from build123d import *

# Parameters (mm, degrees)
HUB_SKETCH_R              = 2.5
HUB_DEPTH                 = 3
POINTER_DEPTH             = 0.8
TAIL_SKETCH_W             = 7.1
TAIL_SKETCH_H             = 3
TAIL_DEPTH                = 3
TAIL_END_SKETCH_R         = 1.5
TAIL_END_DEPTH            = 3
SHAFT_BORE_DEPTH          = 23.343902972
SHAFT_BORE_DEPTH_BACK     = 23.343902972
BORE_SKETCH_R             = 1
SET_SCREW_HOLE_DEPTH      = 23.343902972
SET_SCREW_HOLE_DEPTH_BACK = 23.343902972
SETSCREW_SKETCH_R         = 0.6


with BuildPart() as part:
    # HUB_SKETCH → HUB (new body)
    with BuildSketch(Plane(origin=(0, 0, 0), x_dir=(1, 0, 0), z_dir=(0, 1, 0))):
        with Locations(Location((0, 0, 0), (0, 0, 270))):
            Circle(HUB_SKETCH_R)
    extrude(amount=HUB_DEPTH)

    # POINTER_SKETCH → POINTER (add)
    with BuildSketch(Plane(origin=(0, 0, 0), x_dir=(1, 0, 0), z_dir=(0, 1, 0))):
        Polygon((2, 1.5), (22, 0.3), (22, -0.3), (2, -1.5), align=None)
    extrude(amount=POINTER_DEPTH)

    # TAIL_SKETCH → TAIL (add)
    with BuildSketch(Plane(origin=(0, 0, 0), x_dir=(1, 0, 0), z_dir=(0, 1, 0))):
        with Locations((-3.55, 0)):
            Rectangle(TAIL_SKETCH_W, TAIL_SKETCH_H)
    extrude(amount=TAIL_DEPTH)

    # TAIL_END_SKETCH → TAIL_END (add)
    with BuildSketch(Plane(origin=(0, 0, 0), x_dir=(1, 0, 0), z_dir=(0, 1, 0))):
        with Locations((-7.1, 0)):
            Circle(TAIL_END_SKETCH_R)
    extrude(amount=TAIL_END_DEPTH)

    # BORE_SKETCH → SHAFT_BORE (cut, two sides: drawn at the far end of the back side and taken through both)
    with BuildSketch(Plane(origin=(0, 0, 0), x_dir=(1, 0, 0), z_dir=(0, 1, 0)).offset(-SHAFT_BORE_DEPTH_BACK)):
        with Locations(Location((0, 0, 0), (0, 0, 270))):
            Circle(BORE_SKETCH_R)
    extrude(amount=SHAFT_BORE_DEPTH + SHAFT_BORE_DEPTH_BACK, mode=Mode.SUBTRACT)

    # SETSCREW_SKETCH → SET_SCREW_HOLE (cut, two sides: drawn at the far end of the back side and taken through both)
    with BuildSketch(Plane.XY.offset(-SET_SCREW_HOLE_DEPTH_BACK)):
        with Locations((0, 1.46538664)):
            Circle(SETSCREW_SKETCH_R)
    extrude(amount=SET_SCREW_HOLE_DEPTH + SET_SCREW_HOLE_DEPTH_BACK, mode=Mode.SUBTRACT)


solid = part.part
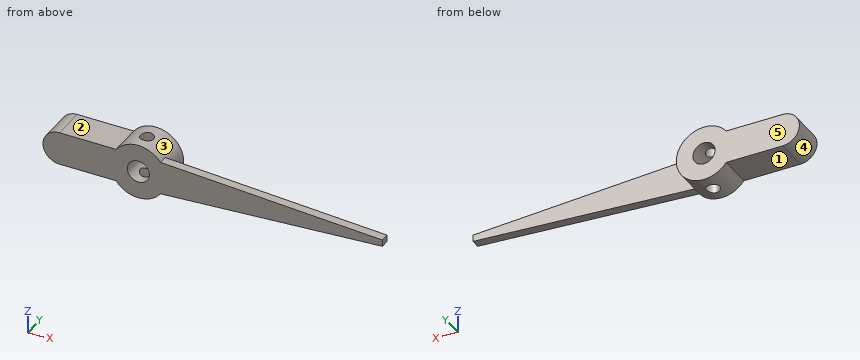
The model under review builds one solid part; all positions refer to its coordinate system, in mm. Face numbers are marked on the shaded views. A direction names the side the tool comes from. Round coordinates to 2 decimals unless told otherwise and drop trailing zeros. Order: outer loops, then holes, each group sorted by start corner. A loop starts at its lowest first (then second) coordinate and runs counter-clockwise, first axis right, second up. Notation, with made-up numbers: (85, 60) - (139, 60) arc R24 cw to (139, 84) - close; hole circle Ø5 at (62, -36.75). An arc over 180 degrees is marked (long way). Use one line per item in the form item = value.
Q1. Add section B-B on z = 0. Give the boundary of the cut face in (x, y), then the cut area to 3 significant figures.
Response values:
outline = (-8.6, 0) - (-1, 0) - (-1, 3) - (-8.6, 3) - close; (1, 0) - (22, 0) - (22, 0.8) - (2.5, 0.8) - (2.5, 3) - (1, 3) - close
area = 42.9 mm^2
Q2. Tool access review of the marked faces 1, 2, 3, 4 and 5: name each direction out of +Z, -Z, +X, -X, +Y, -Y from which nothing blocks a thin tool from reaching the whole face with its end or side.
Response values:
face_1 = -Z, -X, +Y, -Y
face_2 = +Z, -X, +Y, -Y
face_3 = +Y
face_4 = -X, +Y, -Y
face_5 = +Z, -Z, +X, -X, +Y
Q3. To check wall thickness, follow line 1 (Y direction, x = 0, z = -1.4); line 2 (X direction, y = 1.05, z = 0); line 3 (X direction, y = 0.4, z = -0.05). State the ranges of each line that lie inside material, in increasing order.
Response values:
line_1 = 0 to 0.87, 2.07 to 3
line_2 = -8.6 to -1, 1 to 2.5
line_3 = -8.6 to -1, 1 to 22
Q4. Clearance check with flat-ended pins moving along their axes: P1, Ø1.5, axis at y = 2.5, z = -1, coming from the +X side; P2, Ø1.1, axis at x = 0, y = 1.47, coming from the +Z side; P3, Ø1.5, axis at x = 13, z = 0, coming from the +Y side. State where each tip first meets the part, or that it passes through.
Response values:
P1 = 2.49
P2 = through
P3 = 0.8
Q5. Add section D-D on z = 1.85. Give the boundary of the cut face in (x, y), then the cut area to 3 significant figures.
Response values:
outline = (-1.68, 0) - (1.68, 0) - (1.68, 3) - (-1.68, 3) - close; hole circle Ø1.2 at (0, 1.47)
area = 8.96 mm^2
Q6. Add section A-A on x = 0. Give the boundary of the cut face in (y, z), then the cut area to 3 significant figures.
Response values:
outline = (0, -2.5) - (0.87, -2.5) - (0.87, -1) - (0, -1) - close; (0, 1) - (0.87, 1) - (0.87, 2.5) - (0, 2.5) - close; (2.07, -2.5) - (3, -2.5) - (3, -1) - (2.07, -1) - close; (2.07, 1) - (3, 1) - (3, 2.5) - (2.07, 2.5) - close
area = 5.40 mm^2
Q7. Add section C-C on y = 0.5. Give the boundary of the cut face in (x, z), then the cut area to 3 significant figures.
Response values:
outline = (-7.1, -1.5) - (-2, -1.5) arc R2.5 ccw to (2, -1.5) - (22, -0.3) - (22, 0.3) - (2, 1.5) arc R2.5 ccw to (-2, 1.5) - (-7.1, 1.5) arc R1.5 ccw to start; hole circle Ø2 at (0, 0)
area = 69.3 mm^2
